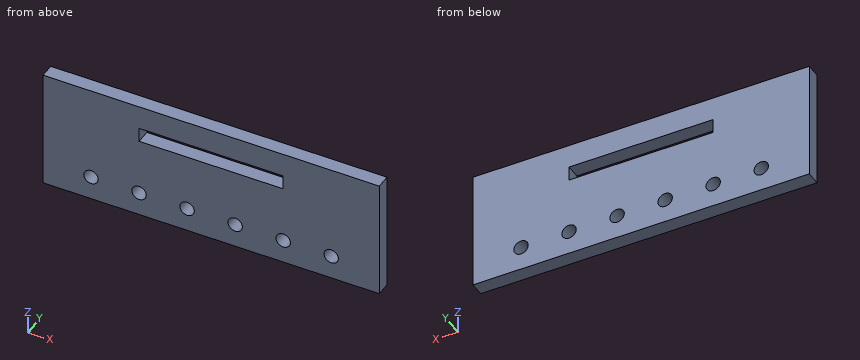
from build123d import *

# Parameters (mm, degrees)
SKETCH1_W           = 70
SKETCH1_H           = 25
SKETCH1_R           = 1.5
SKETCH1_W_2         = 30
SKETCH1_H_2         = 3
BOSS_EXTRUDE1_DEPTH = 3


with BuildPart() as part:
    # Sketch1 → Boss-Extrude1 (new body)
    with BuildSketch(Plane(origin=(0, 0, 0), x_dir=(1, 0, 0), z_dir=(0, 1, 0))):
        Rectangle(SKETCH1_W, SKETCH1_H)
        with Locations(Location((-25, 7.5, 0), (0, 0, 270))):
            Circle(SKETCH1_R, mode=Mode.SUBTRACT)
        with Locations(Location((-15, 7.5, 0), (0, 0, 270))):
            Circle(SKETCH1_R, mode=Mode.SUBTRACT)
        with Locations(Location((-5, 7.5, 0), (0, 0, 270))):
            Circle(SKETCH1_R, mode=Mode.SUBTRACT)
        with Locations(Location((5, 7.5, 0), (0, 0, 270))):
            Circle(SKETCH1_R, mode=Mode.SUBTRACT)
        with Locations(Location((15, 7.5, 0), (0, 0, 270))):
            Circle(SKETCH1_R, mode=Mode.SUBTRACT)
        with Locations(Location((25, 7.5, 0), (0, 0, 270))):
            Circle(SKETCH1_R, mode=Mode.SUBTRACT)
        with Locations((0, -6)):
            Rectangle(SKETCH1_W_2, SKETCH1_H_2, mode=Mode.SUBTRACT)
    extrude(amount=BOSS_EXTRUDE1_DEPTH)


solid = part.part
Can you work these out from the model? Positions are in its coordinate system, mm. Round coordinates to 2 decimals unless told otherwise and drop trailing zeros. Write each loop counter-clockwise with the first axis right and the second up, starting at its lowest first coordinate (ties: lowest second). Pieces come first, ordered by that corner, then holes. Notation, with made-up numbers: M 34.5,75 L 89.5,75 A13 ccw 89.5,96 Z; hole C -8.75,-17 d5. An arc over 180 degrees is marked long. Use a Markdown table: item, result.
Item 1: If I drill on line 1 along X through (y, z) = (1.85, 7.25); line 2 along Z through (x, y) = (-14.5, 1.65); line 3 along Z through (x, y) = (2, 1.2), over which ranges is the centre line in solid material (lowest first)? Write a range as [from, to].
Found:
| item | result |
|---|---|
| line 1 | x = [-35, -15], [15, 35] |
| line 2 | z = [-12.5, -8.91], [-6.09, 4.5], [7.5, 12.5] |
| line 3 | z = [-12.5, 4.5], [7.5, 12.5] |
Item 2: I want a section at B-B (z = -7.5). List the corners of the cut face in (x, y) for me.
Found:
| item | result |
|---|---|
| outline | M -35,0 L -26.5,0 L -26.5,3 L -35,3 Z; M -23.5,0 L -16.5,0 L -16.5,3 L -23.5,3 Z; M -13.5,0 L -6.5,0 L -6.5,3 L -13.5,3 Z; M -3.5,0 L 3.5,0 L 3.5,3 L -3.5,3 Z; M 6.5,0 L 13.5,0 L 13.5,3 L 6.5,3 Z; M 16.5,0 L 23.5,0 L 23.5,3 L 16.5,3 Z; M 26.5,0 L 35,0 L 35,3 L 26.5,3 Z |
Item 3: I want a section at C-C (x = -5). List the corners of the cut face in (y, z) for me.
Found:
| item | result |
|---|---|
| outline | M 0,-12.5 L 3,-12.5 L 3,-9 L 0,-9 Z; M 0,-6 L 3,-6 L 3,4.5 L 0,4.5 Z; M 0,7.5 L 3,7.5 L 3,12.5 L 0,12.5 Z |
Item 4: I want a section at A-A (x = 25). List the corners of the cut face in (y, z) for me.
Found:
| item | result |
|---|---|
| outline | M 0,-12.5 L 3,-12.5 L 3,-9 L 0,-9 Z; M 0,-6 L 3,-6 L 3,12.5 L 0,12.5 Z |
Item 5: I want a section at D-D (y = 0.85). List the corners of the cut face in (x, z) for me, and give its area (3 significant figures).
Found:
| item | result |
|---|---|
| outline | M -35,-12.5 L 35,-12.5 L 35,12.5 L -35,12.5 Z; hole C -25,-7.5 d3; hole C -15,-7.5 d3; hole M -15,4.5 L 15,4.5 L 15,7.5 L -15,7.5 Z; hole C -5,-7.5 d3; hole C 5,-7.5 d3; hole C 15,-7.5 d3; hole C 25,-7.5 d3 |
| area | 1,620 mm2 |
Item 6: For pin 1 Ø4 at (x, z) = (25, -7.5) entering from -Y, with a flat end and sliding along its axis, tell me the tip position at first contact or that it passes through.
Found:
| item | result |
|---|---|
| pin 1 | stops at y = 0 |
